from build123d import *

# Parameters (mm, degrees)
SKETCH2_W           = 220
SKETCH2_H           = 250
BOSS_EXTRUDE2_DEPTH = 80
SKETCH3_W           = 210
SKETCH3_H           = 240
CUT_EXTRUDE1_DEPTH  = 75
FILLET1_R           = 10
CUT_EXTRUDE2_DEPTH  = 75


with BuildPart() as part:
    # Sketch2 → Boss-Extrude2 (new body)
    with BuildSketch(Plane(origin=(0, 0, 0), x_dir=(1, 0, 0), z_dir=(0, 1, 0))):
        Rectangle(SKETCH2_W, SKETCH2_H)
    extrude(amount=BOSS_EXTRUDE2_DEPTH)

    # Sketch3 → Cut-Extrude1 (cut)
    with BuildSketch(Plane(origin=(0, 80, 0), x_dir=(1, 0, 0), z_dir=(0, 1, 0))):
        Rectangle(SKETCH3_W, SKETCH3_H)
    extrude(amount=-CUT_EXTRUDE1_DEPTH, mode=Mode.SUBTRACT)

    # Fillet1
    fillet1_edges = [part.edges().sort_by_distance(p)[0] for p in [
        (-105, 42.5, 120),
        (-105, 42.5, -120),
        (105, 42.5, -120),
        (105, 42.5, 120),
        (-110, 40, -125),
        (110, 40, -125),
        (110, 40, 125),
        (-110, 40, 125),
    ]]
    fillet(fillet1_edges, radius=FILLET1_R)

    # Sketch4 → Cut-Extrude2 (cut)
    with BuildSketch(Plane.XY.offset(125)):
        with BuildLine():
            Line((-7, 5), (-7, 15))
            ThreePointArc((-7, 15), (0, 22), (7, 15))
            Line((7, 15), (7, 5))
            Line((7, 5), (-7, 5))
        make_face()
    extrude(amount=-CUT_EXTRUDE2_DEPTH, mode=Mode.SUBTRACT)


solid = part.part
The model under review builds one solid part; all positions refer to its coordinate system, in mm. A direction names the side the tool comes from. Round coordinates to 2 decimals unless told otherwise and drop trailing zeros. Order: outer loops, then holes, each group sorted by start corner. A loop starts at its lowest first (then second) coordinate and runs counter-clockwise, first axis right, second up. Notation, with made-up numbers: (-4.75, -6.5) -> (10.25, -6.5) arc R34 ccw to (10.25, 28.5) -> close; hole circle Ø6 at (57.25, 36.25). An arc over 180 degrees is marked (long way). Write item = value, one per line. Start each with the question number.
Item 1: For faces 5 (the face through (106.99, 40.56, 122.15)), 6 (the face through (-1, 43, -120)), 7 (the face through (0, 22, 123)), list the 3-axis set-ups (+Z, -Z, +X, -X, +Y, -Y) from which the entire face can be reached by the end or side of a thin tool; tool diameter is ignored.
Item 2: Clearance check with flat-ended pins moving along their axes: pin 1 Ø4 at (x, z) = (3, -1) entering from +Y; pin 2 Ø5.5 at (y, z) = (12, 122) entering from +X; pin 3 Ø5.5 at (y, z) = (11.5, 123) entering from -X. State where each tip first meets the part, or that it passes through.
Item 3: Consider section C-C on y = 46.5. Write out the cut boundary in (x, z).
Item 4: Mouldability with a two-part tool opening along Z and no side actions: class faces 1 (the face through (-105, 43, 2)), 2 (the face through (-1, 39, -125)), 3 (the face through (-107.15, 40.56, 121.99)), 4 (the face through (110, 39, 2)) as released by +Z, released by -Z, zero draft, split by the parting line, or undercut.
Item 5: Consider section B-B on z = -100.5. Write out the cut boundary in (x, y).
Item 6: For line 1 along X through (y, z) = (23, 18.5); line 2 along Z through (x, y) = (17, 71); line 3 along Y through (x, z) = (-42, -32.5), list the stretches that pass through material, from the lowest coordinate up.
Item 7: Consider section D-D on x = -80. Write out the cut boundary in (y, z).
Item 8: Consider section A-A on x = 0. Write out the cut boundary in (y, z).
Conclusion:
q1.face_5 = +Z, +X, +Y, -Y
q1.face_6 = +Y
q1.face_7 = +Z
q2.pin_1 = 5
q2.pin_2 = 109.05
q2.pin_3 = -108.51
q3.outline = (-110, -115) arc R10 ccw to (-100, -125) -> (100, -125) arc R10 ccw to (110, -115) -> (110, 115) arc R10 ccw to (100, 125) -> (-100, 125) arc R10 ccw to (-110, 115) -> close; hole (-105, -110) arc R10 ccw to (-95, -120) -> (95, -120) arc R10 ccw to (105, -110) -> (105, 110) arc R10 ccw to (95, 120) -> (-95, 120) arc R10 ccw to (-105, 110) -> close
q4.face_1 = undercut
q4.face_2 = released by -Z
q4.face_3 = released by +Z
q4.face_4 = zero draft
q5.outline = (-110, 0) -> (110, 0) -> (110, 80) -> (105, 80) -> (105, 5) -> (-105, 5) -> (-105, 80) -> (-110, 80) -> close
q6.line_1 = -110 to -105, 105 to 110
q6.line_2 = -125 to -120, 120 to 125
q6.line_3 = 0 to 5
q7.outline = (0, -125) -> (80, -125) -> (80, -120) -> (5, -120) -> (5, 120) -> (80, 120) -> (80, 125) -> (0, 125) -> close
q8.outline = (0, -125) -> (80, -125) -> (80, -120) -> (5, -120) -> (5, 125) -> (0, 125) -> close; (22, 120) -> (80, 120) -> (80, 125) -> (22, 125) -> close
